Read the model definition and answer for the solid it produces. Units are mm, in the model's axes. A direction names the side the tool comes from. Coordinates: 2 decimals unless noted, no trailing zeros. Loops run counter-clockwise (first coordinate to the right, second up) from the corner with the lowest first, then second, coordinate; pieces in that order, holes last. Notation, with made-up numbers: (-22.5, 69) -> (1.5, 69) arc R12 ccw to (1.5, 91) -> close; hole circle Ø1 at (34.25, -27). An arc over 180 degrees is marked (long way). Answer in a Markdown table with one row per item.
```python
from build123d import *

# Parameters (mm, degrees)
F0_W      = 60
F0_H      = 40
F1_DEPTH  = 50
F3_W      = 10
F3_H      = 35
F5_DEPTH  = 35
F6_R      = 34.99999
F7_DEPTH  = 12.7
F9_DEPTH  = 40
F10_DEPTH = 50.001
F12_DEPTH = 20.001
F13_W     = 20
F13_H     = 10
F14_DEPTH = 60.001


# Not quite as in the source:
# - a fillet or chamfer is up to 0.001 mm smaller than in the source, because OpenCascade refuses the exact size


with BuildPart() as f1:
    # F0 (on Top) → F1 (new body)
    with BuildSketch(Plane.XY):
        with Locations((30, -20)):
            Rectangle(F0_W, F0_H)
    extrude(amount=F1_DEPTH)

    # F3 (on face) → F5 (cut, through all)
    with BuildSketch(Plane.XY.offset(50)):
        with Locations((15, -22.5)):
            Rectangle(F3_W, F3_H)
    extrude(amount=-F5_DEPTH, mode=Mode.SUBTRACT)

    # F6 (radius 35 in the source; OpenCascade refuses exactly that, so slightly less here)
    f6_edges = [f1.edges().sort_by_distance(p)[0] for p in [
        (15, -5, 15),
    ]]
    fillet(f6_edges, radius=F6_R)

    # F2 (on face) → F7 (cut)
    with BuildSketch(Plane(origin=(0, 0, 0), x_dir=(0, -1, 0), z_dir=(-1, 0, 0))):
        Polygon((40, 50), (20, 50), (40, 40), align=None)
    extrude(amount=-F7_DEPTH, mode=Mode.SUBTRACT)

    # F8 (on face) → F9 (cut, through all)
    with BuildSketch(Plane.YZ.offset(60)):
        Polygon((-40, 30), (-20, 50), (-40, 50), align=None)
    extrude(amount=-F9_DEPTH, mode=Mode.SUBTRACT)

    # F3 (on face) → F10 (cut, through all)
    with BuildSketch(Plane.XY.offset(50)):
        Polygon((45, -20), (30, -40), (60, -40), (60, -10), align=None)
    extrude(amount=-F10_DEPTH, mode=Mode.SUBTRACT)

    # F11 (on face) → F12 (cut, through all)
    with BuildSketch(Plane(origin=(0, 0, 0), x_dir=(-1, 0, 0), z_dir=(0, 1, 0))):
        Polygon((-60, 10), (-45, 50), (-60, 50), align=None)
    extrude(amount=-F12_DEPTH, mode=Mode.SUBTRACT)

    # F13 (on face) → F14 (cut, through all)
    with BuildSketch(Plane(origin=(0, 0, 0), x_dir=(0, -1, 0), z_dir=(-1, 0, 0))):
        with Locations((20, 5)):
            Rectangle(F13_W, F13_H)
    extrude(amount=-F14_DEPTH, mode=Mode.SUBTRACT)


solid = f1.part
```
1. A tool of negligible diameter and unlimited length cuts with its end or side. For faces 1 (the flat face through (30, -28, 42)), 2 (the flat face through (0, -20, 25)), 3 (the flat face through (30, -10, 5)), 4 (the flat face through (10, -23, 33)), 5 (the flat face through (18, -35, 0)), from which of +Z, -Z, +X, -X, +Y, -Y can it reach the whole face along a straight path? Write none if from no direction.
A:
| item | result |
|---|---|
| face 1 | +Z, +X, -Y |
| face 2 | +Z, -Z, -X, +Y, -Y |
| face 3 | -Z, +X, -X |
| face 4 | +Z, -Y |
| face 5 | -Z, +X, -X, +Y, -Y |
2. The mould has two halves that part along X. Classify faces 6 (the flat face through (23, -20, 10)), 7 (the flat face through (52.605, -7.638, 29.72)), 8 (the cylindrical face through (15.07, -15.525, 24.981)): pulls with the +X half, pulls with the -X half, needs draft (parallel to the pull), parting line crosses it, or undercut.
A:
| item | result |
|---|---|
| face 6 | needs draft |
| face 7 | pulls with the +X half |
| face 8 | undercut |
3. Given pin 1 Ø6 at (y, z) = (-29, 31) entering from +X; pin 2 Ø4 at (y, z) = (-33, 42) entering from +X; pin 3 Ø1.5 at (x, y) = (44, -21.5) entering from -Z, each flat-ended and moving along its own axis, determine where each tip first touches the part or whether it passes through.
A:
| item | result |
|---|---|
| pin 1 | stops at x = 40.5 |
| pin 2 | stops at x = 10 |
| pin 3 | stops at z = 10 |
4. A cutting plane is placed at B-B on x = 6. Give the vertices of the cut face in (y, z).
A:
| item | result |
|---|---|
| outline | (-40, 0) -> (-30, 0) -> (-30, 10) -> (-10, 10) -> (-10, 0) -> (0, 0) -> (0, 50) -> (-20, 50) -> (-40, 40) -> close |
5. A cutting plane is placed at A-A on z = 3. Give the vertices of the cut face in (x, y).
A:
| item | result |
|---|---|
| outline | (0, -40) -> (30, -40) -> (37.5, -30) -> (0, -30) -> close; (0, -10) -> (60, -10) -> (60, 0) -> (0, 0) -> close |
6. A cutting plane is placed at D-D on z = 42. Give the vertices of the cut face in (x, y), and give its area (3 significant figures).
A:
| item | result |
|---|---|
| outline | (0, -36) -> (10, -36) -> (10, -5.93) -> (20, -5.93) -> (20, -28) -> (39, -28) -> (45, -20) -> (48, -18) -> (48, 0) -> (0, 0) -> close |
| area | 1,150 mm2 |
7. Find the intervals of material crossed by probe 1 along Y at (x, z) = (19.5, 6.5); probe 2 along Z at (x, y) = (35, -20); probe 3 along X at (y, z) = (-26, 45), in increasing order.
A:
| item | result |
|---|---|
| probe 1 | y = -40 to -30, -10 to 0 |
| probe 2 | z = 10 to 50 |
| probe 3 | x = 0 to 10 |
8. A cutting plane is placed at C-C on y = -2.5. Give the vertices of the cut face in (x, z).
A:
| item | result |
|---|---|
| outline | (0, 0) -> (60, 0) -> (60, 10) -> (45, 50) -> (0, 50) -> close |
